Check sheet for the modelled part. Datum: model origin and axes. Units: mm. A direction names the side the tool comes from. Give positions to 0.01 mm unless a question says otherwise; leave off trailing zeros. Write each loop counter-clockwise with the first axis right and the second up, starting at its lowest first coordinate (ties: lowest second). Pieces come first, ordered by that corner, then holes. Notation, with made-up numbers: M -12,-40 L 7,-40 A23 ccw 7,-6 Z; hole C 53.25,-21 d1. An arc over 180 degrees is marked long. Use CSV: the item, a comma, the result in double quotes. Start each with the question number.
1. Depth check by flat-ended pin: P1, Ø8, axis at y = 1, z = 13, coming from the +X side; P2, Ø12, axis at x = -52.5, z = -21, coming from the -Y side; P3, Ø8.5, axis at x = 3, z = -7, coming from the -Y side; P4, Ø5, axis at x = -41, z = -19.5, coming from the +Y side. Enter the tip coordinate at first touch or a pass-through.
2. Cross-section at B-B, the plane x = -44.45. Enter the section's corners in (y, z) (3 decimals).
3. Access from +Z, -Z, +X, -X, +Y, -Y to the whole of each face (thin tool, end or side, straight path). Record for faces 1 (the face through (-43, 6, 0)), 2 (the face through (-36.824, 9.481, -22.212)), 3 (the face through (0, 0, -13)).
4. Cross-section at D-D, the plane z = 5. Enter the section's corners in (x, y), and give its area (3 significant figures).
5. Mould release check, pull along X, two halves, no side actions. Record for faces 4 (the face through (0, -6.35, -15)), 5 (the face through (-63.5, 6, -31)), 6 (the face through (-41, 6.35, -23)), 7 (the face through (0, 2.54, -13)): +X half, -X half, draft (parallel to the pull), parting line (faces both ways), or undercut.
6. Scan lines: line 1 (Z direction, x = -44.45, y = 2); line 2 (Z direction, x = -44.45, y = 10.5) (3 decimals); line 3 (Y direction, x = -29, z = -53.5). Record each from-to range of solid material in increasing order.
7. Cross-section at A-A, the plane z = -44.45. Enter the section's corners in (x, y) (3 decimals).
from build123d import *

# Parameters (mm, degrees)
F0_R          = 8.255
F1_DEPTH      = 12.7
F0_R_2        = 4.28625
F2_DEPTH      = 6.35
F3_DEPTH      = 12.7
F3_DEPTH_BACK = 6.35
F4_DEPTH      = 2.54


with BuildPart() as f1:
    # F0 (on Front) → F1 (new body)
    with BuildSketch(Plane.XZ):
        with BuildLine():
            ThreePointArc((0, -22.225), (-15.715448, -15.715448), (-22.225, 0))
            Line((-22.225, 0), (-63.5, 0))
            Line((-63.5, 0), (-63.5, -63.5))
            Line((-63.5, -63.5), (0, -63.5))
            Line((0, -63.5), (0, -22.225))
        make_face()
        with Locations((-19.05, -44.45)):
            Circle(F0_R, mode=Mode.SUBTRACT)
        with Locations((-44.45, -19.05)):
            Circle(F0_R, mode=Mode.SUBTRACT)
    extrude(amount=F1_DEPTH)

    # F0 (on Front) → F2 (join)
    with BuildSketch(Plane.XZ):
        with Locations((-44.45, -19.05)):
            Circle(F0_R)
        with Locations((-44.45, -19.05)):
            Circle(F0_R_2, mode=Mode.SUBTRACT)
        with Locations((-19.05, -44.45)):
            Circle(F0_R)
        with Locations((-19.05, -44.45)):
            Circle(F0_R_2, mode=Mode.SUBTRACT)
    extrude(amount=F2_DEPTH)

    # F0 (on Front) → F3 (join, two sides)
    with BuildSketch(Plane.XZ) as f3_sk:
        with BuildLine():
            ThreePointArc((-14.4145, 0), (0, 14.4145), (14.4145, 0))
            ThreePointArc((14.4145, 0), (10.192591, -10.192591), (0, -14.4145))
            Line((0, -14.4145), (0, -22.225))
            ThreePointArc((0, -22.225), (15.715448, -15.715448), (22.225, 0))
            ThreePointArc((22.225, 0), (0, 22.225), (-22.225, 0))
            Line((-22.225, 0), (-14.4145, 0))
        make_face()
        with BuildLine():
            ThreePointArc((0, -14.4145), (-10.192591, -10.192591), (-14.4145, 0))
            Line((-14.4145, 0), (-22.225, 0))
            ThreePointArc((-22.225, 0), (-15.715448, -15.715448), (0, -22.225))
            Line((0, -22.225), (0, -14.4145))
        make_face()
    extrude(amount=F3_DEPTH)
    extrude(f3_sk.sketch, amount=-F3_DEPTH_BACK)

    # F0 (on Front) → F4 (join)
    with BuildSketch(Plane.XZ):
        with BuildLine():
            ThreePointArc((0, -14.4145), (10.192591, -10.192591), (14.4145, 0))
            ThreePointArc((14.4145, 0), (0, 14.4145), (-14.4145, 0))
            Line((-14.4145, 0), (-12.7, 0))
            ThreePointArc((-12.7, 0), (0, 12.7), (12.7, 0))
            ThreePointArc((12.7, 0), (8.980256, -8.980256), (0, -12.7))
            Line((0, -12.7), (0, -14.4145))
        make_face()
        with BuildLine():
            Line((-12.7, 0), (-14.4145, 0))
            ThreePointArc((-14.4145, 0), (-10.192591, -10.192591), (0, -14.4145))
            Line((0, -14.4145), (0, -12.7))
            ThreePointArc((0, -12.7), (-8.980256, -8.980256), (-12.7, 0))
        make_face()
    extrude(amount=F4_DEPTH)


with BuildPart() as f5_1:
    # F5: instance of F1
    add(f1.part.mirror(Plane.XZ))


solid = f5_1.part
Worked answers:
1,P1,"stops at x = 20.32"
1,P2,"stops at y = 0"
1,P3,"passes through"
1,P4,"stops at y = 6.35"
2,outline,"M 0,-63.5 L 12.7,-63.5 L 12.7,-27.305 L 6.35,-27.305 L 6.35,-23.336 L 0,-23.336 Z; M 0,-14.764 L 6.35,-14.764 L 6.35,-10.795 L 12.7,-10.795 L 12.7,0 L 0,0 Z"
3,face 1,"+Z, -X, +Y, -Y"
3,face 2,"+Y"
3,face 3,"-Y"
4,outline,"M -21.66,-6.35 L -13.52,-6.35 L -13.52,0 L -11.67,0 L -11.67,2.54 L -13.52,2.54 L -13.52,12.7 L -21.66,12.7 Z; M 11.67,0 L 13.52,0 L 13.52,-6.35 L 21.66,-6.35 L 21.66,12.7 L 13.52,12.7 L 13.52,2.54 L 11.67,2.54 Z"
4,area,"319 mm^2"
5,face 4,"draft"
5,face 5,"-X half"
5,face 6,"undercut"
5,face 7,"undercut"
6,line 1,"z = -63.5 to -23.34, -14.76 to 0"
6,line 2,"z = -63.5 to -27.305, -10.795 to 0"
6,line 3,"y = 0 to 12.7"
7,outline,"M -63.5,0 L -23.336,0 L -23.336,6.35 L -27.305,6.35 L -27.305,12.7 L -63.5,12.7 Z; M -14.764,0 L 0,0 L 0,12.7 L -10.795,12.7 L -10.795,6.35 L -14.764,6.35 Z"
